Can you work these out from the model? Positions are in its coordinate system, mm. Face numbers are marked on the shaded views. A direction names the side the tool comes from. Give positions to 0.01 mm unless a question says otherwise; leave off trailing zeros. Write each loop counter-clockwise with the first axis right and the second up, starting at its lowest first coordinate (ties: lowest second). Pieces come first, ordered by that corner, then holes. Notation, with made-up numbers: M 10,-36 L 69,-36 A36 cw 69,-1 Z; hole C -29.75,24 d11. An arc over 180 degrees is marked long. Answer as CSV lines item,"result". Start each with the question number.
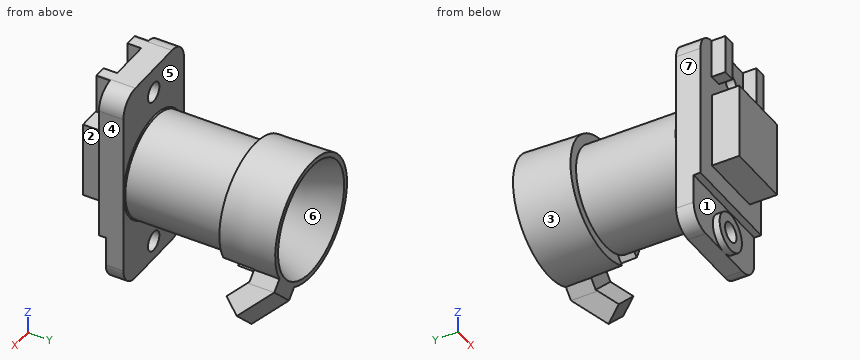
Autodesk Inventor part; units mm, degrees
ref_plane "Work Plane2" through (4.4477, 17.8961, -4.4477) normal (-0.7071, 0, 0.7071) x (0, -1, 0)
ref_plane "YZ Plane" through (0, 0, 0) normal (1, 0, 0) x (0, 1, 0)
ref_plane "XZ Plane" through (0, 0, 0) normal (0, 1, 0) x (-1, 0, 0)
sketch "Sketch1" plane through (0, 0, 0) normal (0, 1, 0) x (-1, 0, 0)
  line L0 (-5.3, -10.5) -> (5.3, -10.5)
  line L1 (5.3, -10.5) -> (5.3, 10.5)
  line L2 (5.3, 10.5) -> (-5.3, 10.5)
  line L3 (-5.3, 10.5) -> (-5.3, -10.5)
  line L4 (-5.3, -10.5) -> (5.3, 10.5) construction
  line L5 (5.3, -10.5) -> (-5.3, 10.5) construction
  point P0 (0, 0)
  dimension "d0" = 10.6
  dimension "d1" = 21
extrude "Extrusion1" add sketch "Sketch1" along normal blind 1.8
sketch "Sketch2" plane through (0, 0, 0) normal (0, -1, 0) x (1, 0, 0)
  line L0 (5.3, -10.5) -> (-5.3, -10.5)
  line L1 (5.3, 10.5) -> (5.3, -10.5)
  line L2 (-5.3, 10.5) -> (5.3, 10.5)
  line L3 (-5.3, -10.5) -> (-5.3, 10.5)
  line L4 (5.3, 10.5) -> (5.3, -10.5)
  line L5 (5.3, -5.4) -> (-5.3, -5.4)
  line L6 (-5.3, -10.5) -> (-5.3, 10.5)
  point P0 (0, 0)
  dimension "d4" = 15.9
extrude "Extrusion2" add sketch "Sketch2" along normal blind 0.7 contours L5 L3 L2 L1
sketch "Sketch3" plane through (0, -0.7, 0) normal (0, -1, 0) x (1, 0, 0)
  line L0 (5.3, 10.5) -> (-5.3, 10.5)
  line L1 (-5.3, 10.5) -> (-5.3, -5.4)
  line L2 (-5.3, -5.4) -> (5.3, -5.4)
  line L3 (5.3, -5.4) -> (5.3, 10.5)
  line L4 (-5.3, 10.5) -> (5.3, 10.5)
  line L5 (3.35, 10.5) -> (2.1, 10.5)
  line L6 (2.1, 10.5) -> (2.1, 6.5)
  line L7 (2.1, 6.5) -> (3.35, 6.5)
  line L8 (3.35, 6.5) -> (3.35, 10.5)
  line L9 (-2.1, 10.5) -> (-3.35, 10.5)
  line L10 (-3.35, 10.5) -> (-3.35, 6.5)
  line L11 (-3.35, 6.5) -> (-2.1, 6.5)
  line L12 (-2.1, 6.5) -> (-2.1, 10.5)
  line L13 (2.1, 7.4366) -> (-2.1, 7.4366) construction
  line L14 (0, 0) -> (0, 2.1174)
  point P0 (0, 7.4366)
  dimension "d7" = 1.25
  dimension "d8" = 4
  dimension "d9" = 1.25
  dimension "d10" = 4
  dimension "d11" = 4.2
extrude "Extrusion3" add sketch "Sketch3" along normal blind 1.4 contours L8 L7 L6 L0 | L12 L11 L10 L0
sketch "Sketch4" plane through (0, -0.7, 0) normal (0, -1, 0) x (1, 0, 0)
  line L0 (3.3, 4.5) -> (-3.3, 4.5)
  line L1 (-3.3, 4.5) -> (-3.3, -3.3)
  line L2 (-3.3, -3.3) -> (3.3, -3.3)
  line L3 (3.3, -3.3) -> (3.3, 4.5)
  line L4 (0, 0) -> (0, 1.0845)
  line L5 (2.1, 10.5) -> (-2.1, 10.5)
  point P0 (0, 4.5)
  dimension "d14" = 6.6
  dimension "d15" = 7.8
  dimension "d16" = 6
extrude "Extrusion4" add sketch "Sketch4" along normal blind 2.8
sketch "Sketch5" plane through (0, 0, 0) normal (0, -1, 0) x (1, 0, 0)
  circle A0 centre (0, -8.55) radius 1.95
  line L0 (5.3, -10.5) -> (-5.3, -10.5)
  point P0 (0, 0)
  dimension "d19" = 3.9
extrude "Extrusion5" add sketch "Sketch5" along normal up to surface (0.7 mm away)
sketch "Sketch6" plane through (0, -0.7, 0) normal (0, -1, 0) x (1, 0, 0)
  line L0 (3.3, 4.5) -> (3.3, -3.3)
  line L1 (3.3, -3.3) -> (-3.3, -3.3)
  line L2 (-3.3, -3.3) -> (-3.3, 4.5)
  line L3 (-3.3, 4.5) -> (3.3, 4.5)
  line L4 (-3.35, 6.5) -> (-3.35, 10.5)
  line L5 (-3.35, 10.5) -> (-5.3, 10.5)
  line L6 (-5.3, 10.5) -> (-5.3, -5.4)
  line L7 (-5.3, -5.4) -> (5.3, -5.4)
  line L8 (5.3, -5.4) -> (5.3, 10.5)
  line L9 (5.3, 10.5) -> (3.35, 10.5)
  line L10 (3.35, 10.5) -> (3.35, 6.5)
  line L11 (3.35, 6.5) -> (2.1, 6.5)
  line L12 (2.1, 6.5) -> (2.1, 10.5)
  line L13 (2.1, 10.5) -> (-2.1, 10.5)
  line L14 (-2.1, 10.5) -> (-2.1, 6.5)
  line L15 (-2.1, 6.5) -> (-3.35, 6.5)
  circle A0 centre (0, -8.55) radius 1.95
  point P0 (0, 0)
  point P1 (0, 7.95)
  dimension "d22" = 16.5
hole "Hole1" at (0, -0.7, 7.95) at (0, -0.7, -8.55) direction (0, 1, 0) diameter 2 end through all
fillet "Fillet1" radius 2.1 4 edges at (-5.3, 0.55, 10.5) (5.3, 0.55, 10.5) (5.3, 0.9, -10.5) (-5.3, 0.9, -10.5)
sketch "Sketch7" plane through (0, 1.8, 0) normal (0, 1, 0) x (1, 0, 0)
  circle A0 centre (0, 0) radius 5.175
  dimension "d31" = 10.35
extrude "Extrusion6" add sketch "Sketch7" along normal blind 10.3
sketch "Sketch8" plane through (0, 0, 0) normal (1, 0, 0) x (0, 1, 0)
  line L0 (12.1, -5.175) -> (12.1, 5.175)
  line L1 (1.8, 5.175) -> (1.8, -5.175)
  line L2 (12.1, -5.175) -> (12.1, 5.175)
  line L3 (12.1, -5.175) -> (12.1, -6.15)
  line L4 (12.1, -6.15) -> (17.8961, -6.29)
  line L5 (17.8961, -6.29) -> (17.8961, -5.79)
  line L6 (17.8961, 0) -> (12.1, 0)
  line L7 (17.8961, -5.79) -> (13.2961, -3.5781)
  line L8 (13.2961, -3.5781) -> (13.2961, 0)
  point P0 (0, 0)
  dimension "d34" = 12.3
  dimension "d35" = 12.58
  dimension "d37" = 2.6
  dimension "d38" = 4.6
  dimension "d39" = 0.5
revolve "Revolution1" add sketch "Sketch8" angle 360 about axis through (0, 17.8961, 0) along (0, -1, 0)
chamfer "Chamfer1" distance 0.12 angle 45 1 edges at (-5.175, 1.8, 0)
sketch "Sketch9" plane through (0, 17.8961, 0) normal (0, 1, 0) x (1, 0, 0)
  line L0 (0, 0) -> (4.9828, 4.9828) construction
  line L1 (0, 0) -> (0, 2.6372) construction
  dimension "d43" = 45
ref_plane "Work Plane2" through (4.4477, 17.8961, -4.4477) normal (-0.7071, 0, 0.7071) x (0, -1, 0)
sketch "Sketch11" plane through (4.4477, 17.8961, -4.4477) normal (-0.7071, 0, 0.7071) x (0, -1, 0)
  line L0 (0, -6.29) -> (0, 6.29)
  line L1 (5.7961, -6.15) -> (5.7961, 6.15)
  line L2 (5.7961, 5.175) -> (5.7961, -5.175)
  line L3 (5.7961, 1.825) -> (2.6, 1.825)
  line L4 (2.6, 1.825) -> (2.6, -1.825)
  line L5 (2.6, -1.825) -> (5.7961, -1.825)
  line L6 (5.7961, -1.825) -> (5.7961, 1.825)
  line L7 (0, 0) -> (0.8817, 0)
  point P0 (17.8961, 0)
  point P1 (2.6, 0)
  dimension "d45" = 3.65
  dimension "d46" = 2.6
extrude "Extrusion7" cut sketch "Sketch11" along normal blind 3.3
sketch "Sketch12" plane through (4.4477, 17.8961, -4.4477) normal (-0.7071, 0, 0.7071) x (0, -1, 0)
  line L0 (5.7961, 1.825) -> (2.6, 1.825)
  line L1 (2.6, 1.825) -> (2.6, -1.825)
  line L2 (2.6, -1.825) -> (5.7961, -1.825)
  line L3 (5.7961, 1.825) -> (5.7961, -1.825)
  line L4 (0, -6.29) -> (0, 6.29)
  line L5 (0, -6.29) -> (0, 6.29)
  line L6 (2.6, 1.825) -> (0, 1.825)
  line L7 (0, 1.825) -> (0, -1.825)
  line L8 (0, -1.825) -> (2.6, -1.825)
  line L9 (2.6, -1.825) -> (2.6, 1.825)
  point P0 (17.8961, 0)
extrude "Extrusion8" add sketch "Sketch12" along normal blind 0.3 and the other way blind 1 contours L1 L8 L4 L6
sketch "Sketch13" plane through (6.4453, 15.2961, -3.8643) normal (0.7071, 0, 0.7071) x (0.7071, 0, -0.7071)
  line L0 (-1.3, 0) -> (-1.3, 1.4344)
  line L1 (-1.3, 0) -> (0, 0)
  line L2 (0, 2.6) -> (0, 0)
  line L3 (0, 2.6) -> (-1.2706, 2.6)
  line L4 (0, 2.6) -> (-1.2706, 2.6)
  line L5 (0, 2.6) -> (3.0642, 0.0288)
  line L6 (3.0642, 0.0288) -> (1.7143, -1.5798)
  line L7 (1.7143, -1.5798) -> (-0.1685, 0)
  line L8 (-1.3, 0) -> (0, 0)
  point P0 (-7.29, -15.2961)
  dimension "d53" = 2.6
  dimension "d54" = 2.1
  dimension "d55" = 40
  dimension "d56" = 4
extrude "Extrusion9" add sketch "Sketch13" against normal up to surface (3.65 mm away)
properties part number "xtion_projector" material "Thermoplastic Resin"
1) I want a section at A-A, the plane y = 1.25. Please give me the cut outline in (x, z), then the cut area to 3 significant figures.
2) On a 3-axis mill with a long thin cutter (end or side, diameter ignored), from which of +Z, -Z, +X, -X, +Y, -Y can I reach the whole of each face in a straight line? I mean the marked faces 1, 2, 3 and 4. Say none if no direction works.
3) I need wall thicknesses on L1, parallel to Z at x = 0, y = 0.4; L2, parallel to X at y = 0.75, z = 7.95; L3, parallel to Y at x = 0.25, z = -6. Which ranges of each line are inside material? Lowest first, please. Write a range as from..to.
4) I want a section at B-B, the plane z = 7.5. Please give me the cut outline in (x, y).
5) I want a section at C-C, the plane z = 0. Please give me the cut outline in (x, y) (3 decimals).
6) Thinking about a two-plate mould opening in Y: for the marked faces 5, 6 and 7, which applies, released by +Y, released by -Y, zero draft, split by the parting line, or undercut?
7) I'm going to push flat-ended pins straight in: P1, Ø1, axis at x = 2.5, z = 8, coming from the -Y side; P2, Ø6, axis at y = 15.5, z = 2.5, coming from the -X side; P3, Ø3, axis at x = 6, y = 0.5, coming from the +Z side. Where does each tip first touch, or does it pass through?
Values found:
1,outline,"M -5.3,-8.4 A2.1 ccw -3.2,-10.5 L 3.2,-10.5 A2.1 ccw 5.3,-8.4 L 5.3,8.4 A2.1 ccw 3.2,10.5 L -3.2,10.5 A2.1 ccw -5.3,8.4 Z; hole C 0,-8.55 d2; hole C 0,7.95 d2"
1,area,"213 mm²"
2,face 1,"-Y"
2,face 2,"-Z, +X, -Y"
2,face 3,"none"
2,face 4,"+Z, -Z, +X, -Y"
3,L1,"z = -10.5..-9.55, -7.55..6.95, 8.95..10.5"
3,L2,"x = -5.3..-1, 1..5.3"
3,L3,"y = 0..1.8, 12.1..17.9"
4,outline,"M -5.3,-0.7 L -3.35,-0.7 L -3.35,-2.1 L -2.1,-2.1 L -2.1,-0.7 L -0.89,-0.7 L -0.89,1.8 L -5.3,1.8 Z; M 0.89,-0.7 L 2.1,-0.7 L 2.1,-2.1 L 3.35,-2.1 L 3.35,-0.7 L 5.3,-0.7 L 5.3,1.8 L 0.89,1.8 Z"
5,outline,"M -6.29,17.896 L -6.15,12.1 L -5.175,12.1 L -5.175,1.92 L -5.295,1.8 L -5.3,1.8 L -5.3,-0.7 L -3.3,-0.7 L -3.3,-3.5 L 3.3,-3.5 L 3.3,-0.7 L 5.3,-0.7 L 5.3,1.8 L 5.295,1.8 L 5.175,1.92 L 5.175,12.1 L 6.15,12.1 L 6.29,17.896 L 5.79,17.896 L 3.578,13.296 L -3.578,13.296 L -5.79,17.896 Z"
6,face 5,"undercut"
6,face 6,"released by +Y"
6,face 7,"zero draft"
7,P1,"stops at y = -2.1"
7,P2,"stops at x = -6.28"
7,P3,"stops at z = 10.05"
